Autodesk Inventor part; units mm, degrees
ref_plane "YZ Plane" through (0, 0, 0) normal (1, 0, 0) x (0, 1, 0)
ref_plane "XZ Plane" through (0, 0, 0) normal (0, 1, 0) x (-1, 0, 0)
ref_plane "XY Plane" through (0, 0, 0) normal (0, 0, 1) x (1, 0, 0)
sketch "Skizze_Grundkörper" plane through (0, 0, 0) normal (0, 0, 1) x (1, 0, 0)
  line L0 (-56, 0) -> (56, 0)
  line L1 (0, -45.5) -> (0, 45.5)
  line L2 (40, -32.5) -> (-40, -32.5)
  line L3 (-40, -32.5) -> (-40, 32.5)
  line L4 (-40, 32.5) -> (40, 32.5)
  line L5 (40, 32.5) -> (40, -32.5)
  line L6 (40, -32.5) -> (-40, 32.5) construction
  line L7 (-40, -32.5) -> (40, 32.5) construction
  point P0 (0, 0)
  dimension "Länge" = 80
  dimension "Höhe" = 65
extrude "Grundkörper" add sketch "Skizze_Grundkörper" along normal blind 10
sketch "Skizze2" plane through (0, 0, 10) normal (0, 0, 1) x (1, 0, 0)
  line L0 (-40, -32.5) -> (40, -32.5)
  line L1 (40, -32.5) -> (40, 32.5)
  line L2 (40, 32.5) -> (-40, 32.5)
  line L3 (-40, 32.5) -> (-40, -32.5)
  line L4 (-56, 0) -> (56, 0)
  line L5 (0, -45.5) -> (0, 45.5)
  point P0 (0, 0)
  point P1 (0, 17.5)
  dimension "d4" = 50
hole "Bohrung_9,7_mm" at (0, 17.5, 10) direction (0, 0, -1) diameter 9.7 end through all
sketch "Skizze3" plane through (0, 0, 10) normal (0, 0, 1) x (1, 0, 0)
  circle A0 centre (0, 17.5) radius 4.85
  line L0 (-40, -32.5) -> (40, -32.5)
  line L1 (40, -32.5) -> (40, 32.5)
  line L2 (40, 32.5) -> (-40, 32.5)
  line L3 (-40, 32.5) -> (-40, -32.5)
  line L4 (-56, 0) -> (56, 0)
  line L5 (0, -45.5) -> (0, 45.5)
  point P0 (0, 0)
  point P1 (-30, -26.5)
  point P2 (30, -26.5)
  dimension "d12" = 60
  dimension "d13" = 6
hole "Bohrung_5,5_mm" at (-30, -26.5, 10) at (30, -26.5, 10) direction (0, 0, -1) diameter 5.5 end through all
chamfer "Fase_10_mm" distance 10 angle 45 2 edges at (-40, 32.5, 5) (40, 32.5, 5)
properties part number "Werkstück_B" material "Stahl, unlegiert"
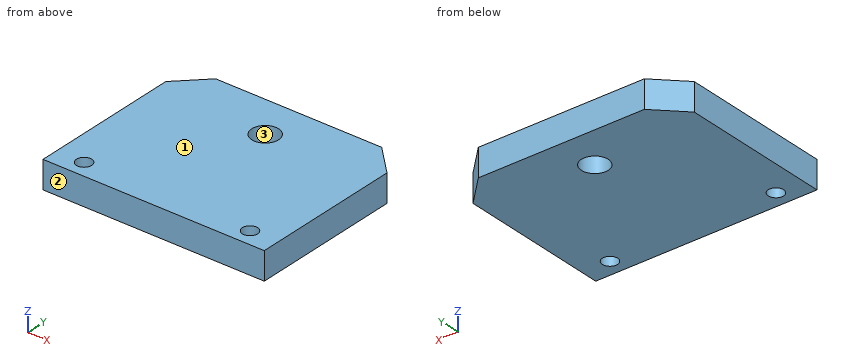
Model file for the job. Use its own axes, mm. Face numbers are marked on the shaded views. Coordinates: 2 decimals unless noted, no trailing zeros. Write each loop counter-clockwise with the first axis right and the second up, starting at its lowest first coordinate (ties: lowest second). Pieces come first, ordered by that corner, then holes. Notation, with made-up numbers: (7.25, 29) - (43.25, 29) arc R18 cw to (43.25, 55) - close; hole circle Ø6 at (19.25, 5). An arc over 180 degrees is marked (long way). One line per question, with ' | ' between items. Start each with the question number.
Q1. Drill centre lines: line 1 (X direction, y = -26.5, z = 4.75); line 2 (X direction, y = 17.5, z = 4.75); line 3 (X direction, y = -27.5, z = 8.75). Where is each one in solid material? Low to high. Write a range as [from, to].
Q2. Cut at C-C, the plane x = 0. List the corners of the cut face in (y, z), then the cut area to 3 significant figures.
Q3. Pull direction Y, two halves, no side cores. Call the marked faces 1, 2 and 3: pulls with the +Y half, pulls with the -Y half, needs draft (parallel to the pull), parting line crosses it, or undercut.
Q4. Cut at D-D, the plane z = 5. List the corners of the cut face in (x, y).
Q5. Cut at B-B, the plane y = 17.5. List the corners of the cut face in (x, z).
Q6. Cut at A-A, the plane y = -26.5. List the corners of the cut face in (x, z).
Answer below:
1) line 1: [-40, -32.75], [-27.25, 27.25], [32.75, 40] | line 2: [-40, -4.85], [4.85, 40] | line 3: [-40, -32.56], [-27.44, 27.44], [32.56, 40]
2) outline: (-32.5, 0) - (12.65, 0) - (12.65, 10) - (-32.5, 10) - close; (22.35, 0) - (32.5, 0) - (32.5, 10) - (22.35, 10) - close | area: 553 mm^2
3) face 1: needs draft | face 2: pulls with the -Y half | face 3: undercut
4) outline: (-40, -32.5) - (40, -32.5) - (40, 22.5) - (30, 32.5) - (-30, 32.5) - (-40, 22.5) - close; hole circle Ø5.5 at (-30, -26.5); hole circle Ø9.7 at (0, 17.5); hole circle Ø5.5 at (30, -26.5)
5) outline: (-40, 0) - (-4.85, 0) - (-4.85, 10) - (-40, 10) - close; (4.85, 0) - (40, 0) - (40, 10) - (4.85, 10) - close
6) outline: (-40, 0) - (-32.75, 0) - (-32.75, 10) - (-40, 10) - close; (-27.25, 0) - (27.25, 0) - (27.25, 10) - (-27.25, 10) - close; (32.75, 0) - (40, 0) - (40, 10) - (32.75, 10) - close
